Geometry: see drawing. Coordinates: mm, zero at the bounding-box minimum. A direction names the side the tool comes from. Coordinates: 2 decimals unless noted, no trailing zeros. Loops run counter-clockwise (first coordinate to the right, second up) from the corner with the lowest first, then second, coordinate; pieces in that order, holes last. Notation, with made-up numbers: (24, -38) -> (46, -38) arc R32 cw to (46, -4) -> close; hole circle Ø7 at (17.25, 85). An arc over 180 degrees is marked (long way). Answer as a JSON object with one key per item and string values.
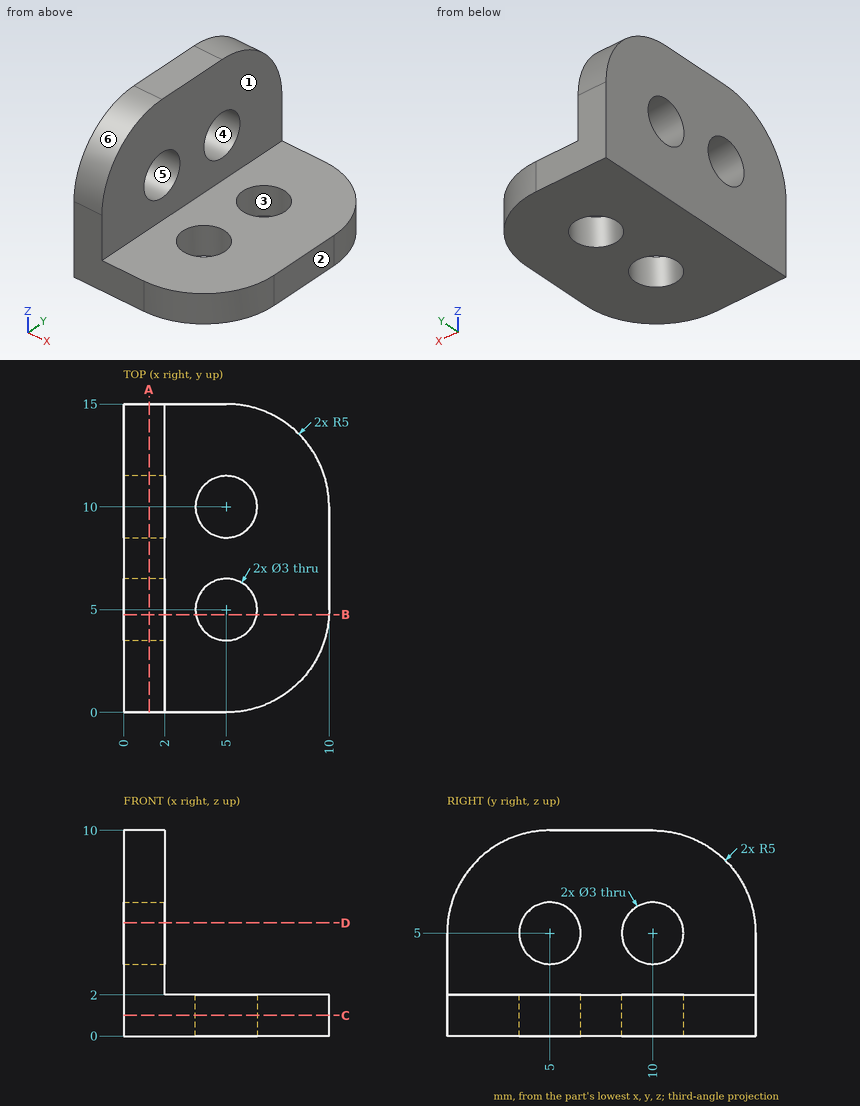
1. Section query D-D (z = 5.5). Return loops of the section in (x, y).
Reply:
{"outline": "(0, 0.03) -> (2, 0.03) -> (2, 3.59) -> (0, 3.59) -> close; (0, 6.41) -> (2, 6.41) -> (2, 8.59) -> (0, 8.59) -> close; (0, 11.41) -> (2, 11.41) -> (2, 14.97) -> (0, 14.97) -> close"}
2. Section query C-C (z = 1). Return loops of the section in (x, y), plus the area to 3 significant figures.
Reply:
{"outline": "(0, 0) -> (5, 0) arc R5 ccw to (10, 5) -> (10, 10) arc R5 ccw to (5, 15) -> (0, 15) -> close; hole circle Ø3 at (5, 5); hole circle Ø3 at (5, 10)", "area": "125 mm2"}
3. Section query A-A (x = 1.25). Return loops of the section in (y, z), plus the area to 3 significant figures.
Reply:
{"outline": "(0, 0) -> (15, 0) -> (15, 5) arc R5 ccw to (10, 10) -> (5, 10) arc R5 ccw to (0, 5) -> close; hole circle Ø3 at (5, 5); hole circle Ø3 at (10, 5)", "area": "125 mm2"}
4. Mould query, pull axis Z, two halves, no side actions, for the marked faces 3, 4, 5 and 6. Classes: pulls with the +Z half, pulls with the -Z half, needs draft (parallel to the pull), parting line crosses it, or undercut.
Reply:
{"face 3": "needs draft", "face 4": "undercut", "face 5": "undercut", "face 6": "pulls with the +Z half"}
5. Pin query (flat end, axial travel): P1, Ø1.5, axis at x = 6, y = 5, coming from the +Z side. Return the tip coordinate at first contact, or that it passes through.
Reply:
{"P1": "stops at z = 2"}
6. Line query: line 1 along Z through (x, y) = (9.75, 9); line 2 along X through (y, z) = (5.5, 1.5). Output: solid intervals per line, ascending.
Reply:
{"line 1": "z = 0 to 2", "line 2": "x = 0 to 3.59, 6.41 to 10"}
7. Section query B-B (y = 4.75). Return loops of the section in (x, z).
Reply:
{"outline": "(0, 0) -> (3.52, 0) -> (3.52, 2) -> (2, 2) -> (2, 3.52) -> (0, 3.52) -> close; (0, 6.48) -> (2, 6.48) -> (2, 9.99) -> (0, 9.99) -> close; (6.48, 0) -> (9.99, 0) -> (9.99, 2) -> (6.48, 2) -> close"}
8. Access query for the marked faces 1 and 2. Directions: +Z, -Z, +X, -X, +Y, -Y. A direction counts if a zero-diameter tool reaches every point of the face in a straight line with its end or side. Return the directions, or none.
Reply:
{"face 1": "+Z, +X, +Y, -Y", "face 2": "+Z, -Z, +X, +Y, -Y"}
